Model file for the job. Use its own axes, mm. Face numbers are marked on the shaded views. Give positions to 0.01 mm unless a question says otherwise; leave off trailing zeros. Write each loop counter-clockwise with the first axis right and the second up, starting at its lowest first coordinate (ties: lowest second). Pieces come first, ordered by that corner, then holes.
```python
from build123d import *

# Parameters (mm, degrees)
CROQUIS1_R              = 8.25
SALIENTE_EXTRUIR1_DEPTH = 5
CROQUIS11_R             = 8.25
SALIENTE_EXTRUIR2_DEPTH = 1
CROQUIS13_W             = 16.491898527
CROQUIS13_H             = 1.592253137
CORTAR_EXTRUIR11_DEPTH  = 25.32457605


with BuildPart() as part:
    # Croquis1 → Saliente-Extruir1 (new body)
    with BuildSketch(Plane(origin=(0, 0, 0), x_dir=(1, 0, 0), z_dir=(0, 1, 0))):
        with Locations(Location((0, 0, 0), (0, 0, 270))):
            Circle(CROQUIS1_R)
    extrude(amount=SALIENTE_EXTRUIR1_DEPTH)

    # Croquis10 → Cortar-Revolución1 (revolve, cut)
    with BuildSketch(Plane(origin=(0, 7.5, 0), x_dir=(1, 0, 0), z_dir=(0, 1, 0))):
        with BuildLine():
            Line((0, 8.25), (0, -8.25))
            ThreePointArc((0, -8.25), (8.25, 0), (0, 8.25))
        make_face()
    revolve(axis=Axis((0, 7.5, -8.25), (0, 0, 1)), mode=Mode.SUBTRACT)

    # Croquis11 → Saliente-Extruir2 (add, symmetric)
    with BuildSketch(Plane(origin=(0, 0, 0), x_dir=(0, 0, -1), z_dir=(1, 0, 0))):
        with Locations((0, 7.5)):
            Circle(CROQUIS11_R)
    extrude(amount=SALIENTE_EXTRUIR2_DEPTH, both=True)

    # Croquis13 → Cortar-Extruir11 (cut, through all)
    with BuildSketch(Plane.XY.offset(-8.35)):
        with Locations((-0.004050736, -0.796126569)):
            Rectangle(CROQUIS13_W, CROQUIS13_H)
    extrude(amount=CORTAR_EXTRUIR11_DEPTH, mode=Mode.SUBTRACT)


solid = part.part
```
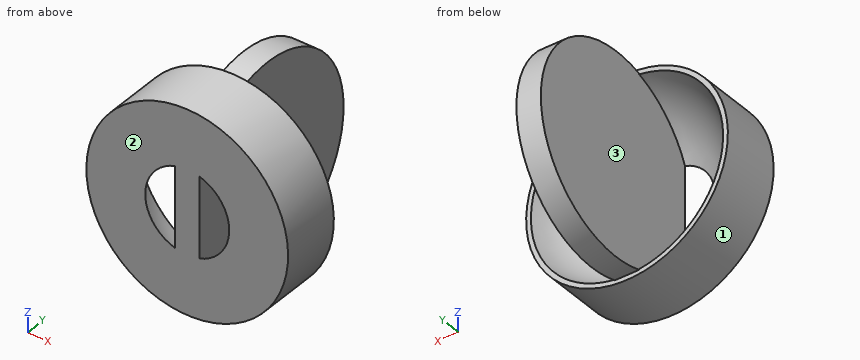
1. Slice it at B-B, the plane z = 0. Write the cut outline in (x, y).
Calculated:
outline: (-8.25, 0) - (-3.44, 0) arc R8.25 cw to (-7.86, 5) - (-8.25, 5) - close; (-1, 0) - (1, 0) - (1, 15.75) - (-1, 15.75) - close; (3.44, 0) - (8.25, 0) - (8.25, 5) - (7.86, 5) arc R8.25 cw to start
2. Slice it at A-A, the plane x = -2. Write the cut outline in (y, z).
Calculated:
outline: (0, -8) - (5, -8) - (5, -7.6) arc R8 cw to (0, -2.8) - close; (0, 2.8) arc R8 cw to (5, 7.6) - (5, 8) - (0, 8) - close
3. Probe probe 1 along X at (y, z) = (4.75, 0); probe 2 along X at (y, z) = (4.25, 3.25); probe 3 along X at (y, z) = (10.5, 0.75). List the from-to ranges inside material, lowest first.
Calculated:
probe 1: x = -8.25 to -7.78, -1 to 1, 7.78 to 8.25
probe 2: x = -7.58 to -6.85, -1 to 1, 6.85 to 7.58
probe 3: x = -1 to 1
4. Slice it at C-C, the plane y = 7.5. Write the cut outline in (x, z), and give its area (3 significant figures).
Calculated:
outline: (-1, -8.25) - (1, -8.25) - (1, 8.25) - (-1, 8.25) - close
area: 33.0 mm2
5. Slice it at D-D, the plane x = 0. Write the cut outline in (y, z).
Calculated:
outline: (0, -8.25) - (5, -8.25) - (5, -7.86) arc R8.25 ccw (long way) to (5, 7.86) - (5, 8.25) - (0, 8.25) - close
6. Pin check, flat tips, straight feed: P1, Ø2, axis at y = 14, z = 0, coming from the +X side; P2, Ø6, axis at x = -4.5, z = 2.5, coming from the -Y side; P3, Ø1, axis at y = 12, z = -4.5, coming from the -X side; P4, Ø8, axis at y = 8.5, z = 2.5, coming from the +X side. Stop position of each tip, or through.
Calculated:
P1: stops at x = 1
P2: stops at y = 0
P3: stops at x = -1
P4: stops at x = 8.23
7. Pull direction X, two halves, no side cores. Call the marked faces 1, 2 and 3: +X half, -X half, draft (parallel to the pull), parting line (faces both ways), or undercut.
Calculated:
face 1: parting line
face 2: draft
face 3: undercut
